The listing builds one solid part. Answer for the finished solid, in the listing's coordinates (mm). Face numbers are marked on the shaded views. Give positions to 0.01 mm unless a question says otherwise; leave off trailing zeros. Loops run counter-clockwise (first coordinate to the right, second up) from the corner with the lowest first, then second, coordinate; pieces in that order, holes last. Notation, with made-up numbers: (31, -4) - (38, -4) arc R29 ccw to (38, 26) - close; hole circle Ø11 at (-31.75, -6.5). An arc over 180 degrees is marked (long way). Write each question's results on one line, items separated by ' | '.
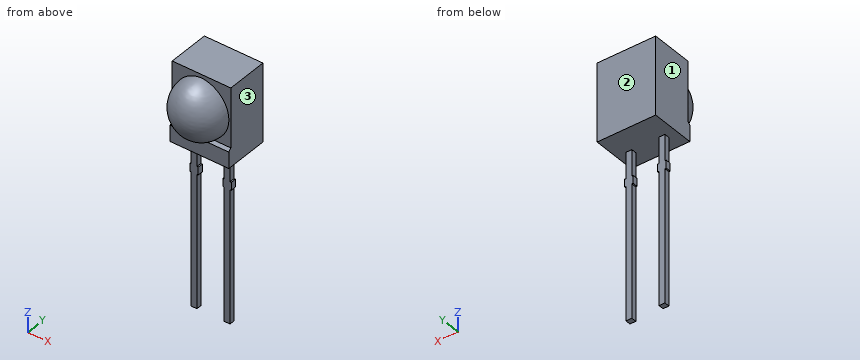
Autodesk Inventor part; units mm, degrees
ref_plane "Arbeitsebene1" through (-2.25, 0.9, -3.5) normal (0, -1, 0) x (1, 0, 0)
ref_plane "YZ Plane" through (0, 0, 0) normal (1, 0, 0) x (0, 1, 0)
ref_plane "XZ Plane" through (0, 0, 0) normal (0, 1, 0) x (-1, 0, 0)
sketch "Skizze3" plane through (0, 0, 0) normal (1, 0, 0) x (0, 1, 0)
  line L0 (3.2, 2.5) -> (0, 2.5)
  line L1 (0, 2.5) -> (0, -2.05)
  line L2 (0, -2.05) -> (-0.2, -2.25)
  line L3 (-0.2, -2.25) -> (-0.2, -3.5)
  line L4 (-0.2, -3.5) -> (3.2, -3.5)
  line L5 (3.2, -3.5) -> (3.2, 2.5)
  line L6 (0, 3.7) -> (0, -4.7)
  line L7 (-0.88, 0) -> (3.88, 0)
  point P0 (0, 0)
  dimension "d5" = 3.2
  dimension "d6" = 6
  dimension "d7" = 2.5
  dimension "d8" = 3.4
  dimension "d9" = 45
  dimension "d10" = 4.55
extrude "Extrusion2" add sketch "Skizze3" along normal mid plane 4.5
sketch "Skizze4" plane through (0, 0, 0) normal (1, 0, 0) x (0, 1, 0)
  line L0 (0, -2.05) -> (0, 2.5)
  arc A0 (0, 2.245) -> (0, -2.245) centre (0.15, 0) ccw
  line L1 (3.2, 2.5) -> (0, 2.5)
  line L2 (0, 2.245) -> (0, -2.245)
  point P0 (0, 0)
  dimension "d13" = 2.25
  dimension "d14" = 0.15
  dimension "d15" = 2.5
revolve "Umdrehung1" add sketch "Skizze4" angle 180 mid plane about axis through (0, 0, -2.05) along (0, 0, 1)
ref_plane "Arbeitsebene1" through (-2.25, 0.9, -3.5) normal (0, -1, 0) x (1, 0, 0)
sketch "Skizze5" plane through (-2.25, 0.9, -3.5) normal (0, -1, 0) x (1, 0, 0)
  line L0 (0.755, 0) -> (1.205, 0)
  line L1 (1.205, -12.8) -> (0.755, -12.8)
  line L2 (0, 0) -> (4.5, 0)
  line L3 (1.305, -2) -> (1.305, -2.6)
  line L4 (0.655, -2.6) -> (0.655, -2)
  line L5 (0.655, -2) -> (0.755, -2)
  line L6 (1.205, -2) -> (1.305, -2)
  line L7 (1.305, -2.6) -> (1.205, -2.6)
  line L8 (0.755, -2.6) -> (0.655, -2.6)
  line L9 (0.755, -12.8) -> (0.755, -2.6)
  line L10 (0.755, -2) -> (0.755, 0)
  line L11 (1.205, 0) -> (1.205, -2)
  line L12 (1.205, -2.6) -> (1.205, -12.8)
  line L13 (0.98, -12.8) -> (0.98, 0) construction
  line L14 (4.5, 6) -> (0, 6) construction
  point P0 (2.25, 3.5)
  dimension "d18" = 0.45
  dimension "d19" = 0.65
  dimension "d20" = 0.6
  dimension "d21" = 8.6
  dimension "d22" = 18.8
  dimension "d23" = 1.27
extrude "Extrusion3" add sketch "Skizze5" against normal blind 0.4
mirror "Spiegeln1" about plane through (0, 0, 0) normal (1, 0, 0) of "Extrusion3"
properties part number "Fotodiode BPV23F"
Item 1: A cutting plane is placed at A-A, the plane z = -3.75. Determine the outline of the cut face in (x, y) (3 decimals).
Values found:
outline: (-1.495, 0.9) - (-1.045, 0.9) - (-1.045, 1.3) - (-1.495, 1.3) - close; (1.045, 0.9) - (1.495, 0.9) - (1.495, 1.3) - (1.045, 1.3) - close
Item 2: Find the intervals of material crossed by line 1 along X through (y, z) = (1.2, -10) (3 decimals); line 2 along Y through (x, z) = (1.45, -2.5); line 3 along X through (y, z) = (-0.3, -1.5), in increasing order. Write a range as [from, to].
Values found:
line 1: x = [-1.495, -1.045], [1.045, 1.495] | line 2: y = [-0.2, 3.2] | line 3: x = [-1.5, 1.5]
Item 3: Flat-ended cylindrical pins translate along their axes: P1, Ø2.5, axis at x = 1, y = 2, coming from the -Z side; P2, Ø1.4, axis at x = -0.5, z = -3, coming from the -Y side. Find the tip coordinate at first contact, or state that the pin passes through.
Values found:
P1: stops at z = -16.3 | P2: stops at y = -0.2
Item 4: A cutting plane is placed at B-B, the plane y = 1.95. Determine the outline of the cut face in (x, z).
Values found:
outline: (-2.25, -3.5) - (2.25, -3.5) - (2.25, 2.5) - (-2.25, 2.5) - close
Item 5: For a pull along X with two mould halves and no side action, classify the marked faces 1, 2 and 3 as released by +X, released by -X, zero draft, split by the parting line, or undercut.
Values found:
face 1: released by -X | face 2: zero draft | face 3: released by +X
